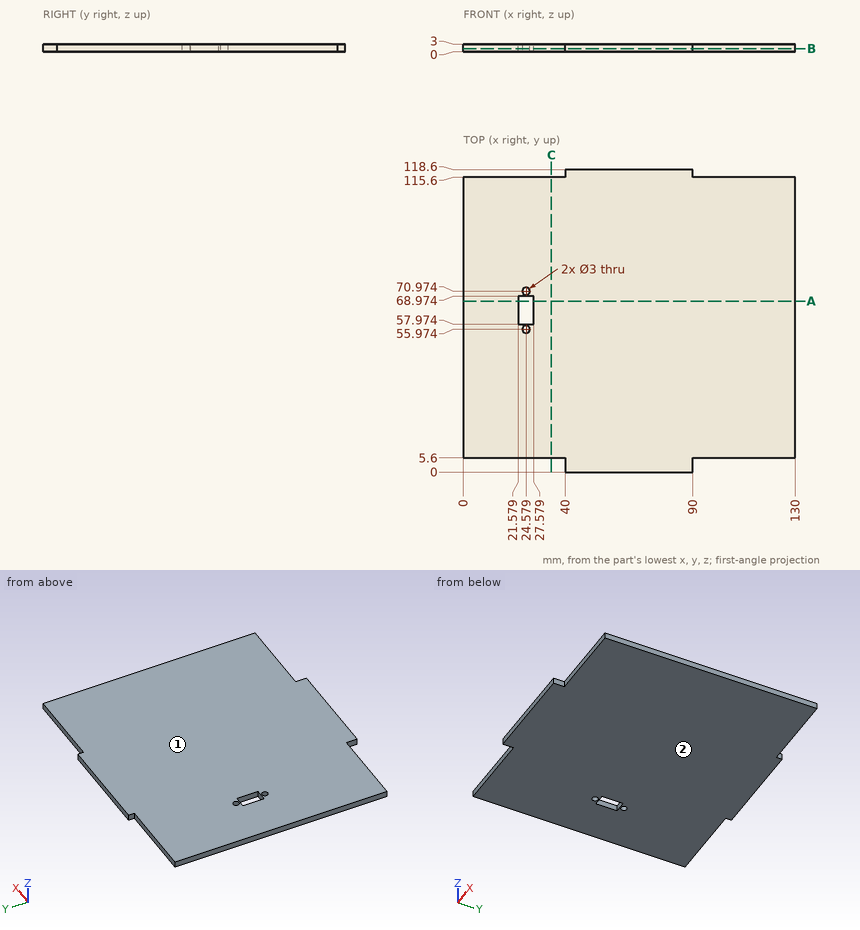
Check sheet for the drawn part. Datum: minimum x, y, z corner. Units: mm. Round coordinates to 2 decimals unless told otherwise and drop trailing zeros. Write each loop counter-clockwise with the first axis right and the second up, starting at its lowest first coordinate (ties: lowest second). Pieces come first, ordered by that corner, then holes. Notation, with made-up numbers: (-3.75, 68.5) - (15.25, 68.5) arc R18 cw to (15.25, 103.5) - close; hole circle Ø1 at (31, 16). An arc over 180 degrees is marked (long way). Return JSON: item names as keys, results as strings.
Q1. Cross-section at B-B (z = 1.2). Record the boundary of the cut face in (x, y).
Returned:
{"outline": "(0, 5.6) - (40, 5.6) - (40, 0) - (90, 0) - (90, 5.6) - (130, 5.6) - (130, 115.6) - (90, 115.6) - (90, 118.6) - (40, 118.6) - (40, 115.6) - (0, 115.6) - close; hole (21.58, 57.97) - (27.58, 57.97) - (27.58, 68.97) - (21.58, 68.97) - close; hole circle Ø3 at (24.58, 55.97); hole circle Ø3 at (24.58, 70.97)"}
Q2. Scan lines: L1, parallel to X at y = 62, z = 0.75; L2, parallel to Y at x = 120.5, z = 1.8; L3, parallel to X at y = 55, z = 2.85. Record each from-to range of solid material in increasing order. Write a range as from..to.
Returned:
{"L1": "x = 0..21.58, 27.58..130", "L2": "y = 5.6..115.6", "L3": "x = 0..23.44, 25.72..130"}
Q3. Draft check along Z on the marked faces 1 and 2. Enter one of: released by +Z, released by -Z, zero draft, split by the parting line, or undercut.
Returned:
{"face 1": "released by +Z", "face 2": "released by -Z"}
Q4. Depth check by flat-ended pin: P1, Ø0.9, axis at y = 116.5, z = 1, coming from the -X side; P2, Ø1, axis at x = 97.5, z = 2.5, coming from the +Y side; P3, Ø1.5, axis at x = 24, z = 1, coming from the -Y side. Enter the tip coordinate at first touch or a pass-through.
Returned:
{"P1": "stops at x = 40", "P2": "stops at y = 115.6", "P3": "stops at y = 5.6"}
Q5. Cross-section at A-A (y = 67). Record the boundary of the cut face in (x, z), then the cut area to 3 significant figures.
Returned:
{"outline": "(0, 0) - (21.58, 0) - (21.58, 3) - (0, 3) - close; (27.58, 0) - (130, 0) - (130, 3) - (27.58, 3) - close", "area": "372 mm²"}
Q6. Cross-section at C-C (x = 34.5). Record the boundary of the cut face in (y, z), then the cut area to 3 significant figures.
Returned:
{"outline": "(5.6, 0) - (115.6, 0) - (115.6, 3) - (5.6, 3) - close", "area": "330 mm²"}
